Geometry check sheet. Reference: the model listing, model coordinates, mm. Face numbers are marked on the shaded views. Coordinates: 2 decimals unless noted, no trailing zeros. Order: outer loops, then holes, each group sorted by start corner. A loop starts at its lowest first (then second) coordinate and runs counter-clockwise, first axis right, second up. Notation, with made-up numbers: (50, 22) - (63, 22) arc R14 cw to (63, 49) - close; hole circle Ø9 at (78, -24.5). An arc over 180 degrees is marked (long way). Use CSV: the item, a comma, the result in double quotes. Start each with the question number.
1) Sectioned sample at D-D, the plane z = 24.75. Record the cut outline in (x, y), and give its area (3 significant figures).
2) Draft check along X on the marked faces 1, 2 and 3. Enter one of: released by +X, released by -X, zero draft, split by the parting line, or undercut.
3) Depth check by flat-ended pin: P1, Ø4, axis at y = -3.5, z = 13.5, coming from the +X side; P2, Ø8, axis at x = -42.5, z = 16.5, coming from the -Y side; P3, Ø8, axis at x = -44.5, y = 0, coming from the +Z side; P4, Ø1, axis at x = -39, y = 0.5, coming from the +Z side. Enter the tip coordinate at first touch or a pass-through.
4) Thickness scan on probe 1 along X at (y, z) = (0, 18.25); probe 2 along Z at (x, y) = (-48.8, 0); probe 3 along X at (y, z) = (0.75, 13). Record the ranges inside material, lowest first. Write a range as [from, to].
5) Sectioned sample at B-B, the plane z = 21.75. Record the cut outline in (x, y).
6) Sectioned sample at C-C, the plane y = -4.5. Record the cut outline in (x, z).
7) Sectioned sample at A-A, the plane y = 0. Record the cut outline in (x, z), and give its area (3 significant figures).
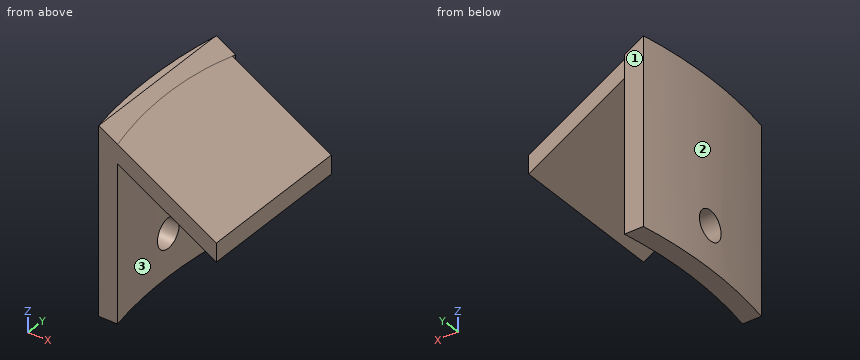
from build123d import *

# Parameters (mm, degrees)
PAD011_DEPTH            = 20
PAD012_DEPTH            = 17
POCKET007_DEPTH         = 17.359799
SKETCH024_R             = 1.6
POCKET008_DEPTH         = 48.751
BODY008_PLACEMENT_ANGLE = 180


with BuildPart() as part:
    # Sketch021 → Pad011 (new body)
    with BuildSketch(Plane.XY):
        with BuildLine():
            ThreePointArc((47.995272, -8.544961), (48.749809, 0.136622), (47.946624, 8.813839))
            Line((45.911641, 8.813839), (47.946624, 8.813839))
            ThreePointArc((45.962443, -8.544961), (46.7498, 0.136818), (45.911641, 8.813839))
            Line((45.962443, -8.544961), (47.995272, -8.544961))
        make_face()
    extrude(amount=PAD011_DEPTH)

    # Sketch022 (on Face1 of Pad011) → Pad012 (join)
    with BuildSketch(Plane.XZ.offset(8.544961)):
        Polygon((47.995272, 0), (35.335121, 7.309342), (35.335121, 9.309342), (47.995272, 2), align=None)
    extrude(amount=-PAD012_DEPTH)

    # Sketch023 (on Face1 of Pad012) → Pocket007 (cut, through all)
    with BuildSketch(Plane.XZ.offset(8.544961)):
        Polygon((43.159527, 2.791919), (47.995272, 0), (43.159527, 0), align=None)
    extrude(amount=-POCKET007_DEPTH, mode=Mode.SUBTRACT)

    # Sketch024 → Pocket008 (cut, through all)
    with BuildSketch(Plane.YZ):
        with Locations((0, 15.434235)):
            Circle(SKETCH024_R)
    extrude(amount=POCKET008_DEPTH, mode=Mode.SUBTRACT)


with BuildPart() as part_1:
    # Body008 placement: moved
    add(part.part.moved(Location((-0.78, 0, 26.9))).rotate(Axis((-0.78, 0, 26.9), (0, 1, 0)), BODY008_PLACEMENT_ANGLE))


solid = part_1.part
Evaluation:
1,outline,"(-48.78, -8.54) - (-45.05, -8.54) - (-45.05, 8.46) - (-46.76, 8.46) arc R46.75 cw to (-46.69, 8.81) - (-48.73, 8.81) arc R48.75 ccw to start"
1,area,"72.6 mm²"
2,face 1,"zero draft"
2,face 2,"released by -X"
2,face 3,"undercut"
3,P1,"x = -47.21"
3,P2,"through"
3,P3,"z = 26.74"
3,P4,"z = 21.54"
4,probe 1,"[-49.53, -47.53], [-37.26, -36.12]"
4,probe 2,"[6.9, 9.87], [13.07, 26.9]"
4,probe 3,"[-49.52, -47.52]"
5,outline,"(-48.78, -8.54) - (-46.74, -8.54) arc R46.75 cw to (-46.69, 8.81) - (-48.73, 8.81) arc R48.75 ccw to start; (-43.32, -8.54) - (-39.86, -8.54) - (-39.86, 8.46) - (-43.32, 8.46) - close"
6,outline,"(-49.32, 6.9) - (-47.31, 6.9) - (-47.31, 24.06) - (-36.12, 17.59) - (-36.12, 19.59) - (-48.78, 26.9) - (-49.32, 26.9) - close"
7,outline,"(-49.53, 6.9) - (-47.53, 6.9) - (-47.53, 9.87) - (-49.53, 9.87) - close; (-49.53, 13.07) - (-47.53, 13.07) - (-47.53, 24.18) - (-36.12, 17.59) - (-36.12, 19.59) - (-48.78, 26.9) - (-49.53, 26.9) - close"
7,area,"56.0 mm²"
